```python
from build123d import *

# Parameters (mm, degrees)
SKETCH1_W                    = 20
SKETCH1_H                    = 85
BASE_FLANGE1_DEPTH           = 1.5
EDGE_FLANGE1_DEPTH           = 85
EDGE_FLANGE2_STRIP_W         = 9
EDGE_FLANGE2_STRIP_H         = 1.5
EDGE_FLANGE2_STRIP_CUT_DEPTH = 85
EDGE_FLANGE2_DEPTH           = 85
CUT_EXTRUDE1_DEPTH           = 53.891398166
CUT_EXTRUDE1_DEPTH_BACK      = 53.891398166
SKETCH13_W                   = 25
SKETCH13_H                   = 26.5
CUT_EXTRUDE2_DEPTH           = 53.891398166
CUT_EXTRUDE2_DEPTH_BACK      = 53.891398166
SKETCH14_W                   = 2.598076211
SKETCH14_H                   = 25
SKETCH15_R                   = 2.25
CAGE_MOUNTING_HOLE_DEPTH     = 53.891398166
EDGE_FLANGE3_DEPTH           = 20
ARDUINO_MOUNTING_HOLE_REACH  = 58.065
SKETCH19_R                   = 1.6
FILLET1_R                    = 2.5


# Sheet-metal steps are written as plain solids
with BuildPart() as part:
    # Sketch1 → Base-Flange1 (new body)
    with BuildSketch(Plane(origin=(0, 0, 0), x_dir=(1, 0, 0), z_dir=(0, 1, 0))):
        Rectangle(SKETCH1_W, SKETCH1_H)
    extrude(amount=-BASE_FLANGE1_DEPTH)

    # Edge-Flange1 section (across the edge) → Edge-Flange1 (add)
    with BuildSketch(Plane(origin=(-11.5, 0, -42.5), x_dir=(1, 0, 0), z_dir=(0, 0, 1))):
        with BuildLine():
            Line((-1.5, 1.5), (-1.5, 25))
            Line((-1.5, 25), (0, 25))
            Line((0, 25), (0, 1.5))
            ThreePointArc((0, 1.5), (0.439339828, 0.439339828), (1.5, 0))
            Line((1.5, 0), (1.5, -1.5))
            ThreePointArc((1.5, -1.5), (-0.621320344, -0.621320344), (-1.5, 1.5))
        make_face()
    extrude(amount=EDGE_FLANGE1_DEPTH)

    # Edge-Flange2 strip (across the edge) → Edge-Flange2 strip cut (cut)
    with BuildSketch(Plane(origin=(-11.5, 25, -42.5), x_dir=(0, -1, 0), z_dir=(0, 0, 1))):
        with Locations((-3, -0.75)):
            Rectangle(EDGE_FLANGE2_STRIP_W, EDGE_FLANGE2_STRIP_H)
    extrude(amount=EDGE_FLANGE2_STRIP_CUT_DEPTH, mode=Mode.SUBTRACT)

    # Edge-Flange2 section (across the edge) → Edge-Flange2 (add)
    with BuildSketch(Plane(origin=(-11.5, 25, -42.5), x_dir=(0, -1, 0), z_dir=(0, 0, 1))):
        with BuildLine():
            Line((-1.5, 1.5), (-1.5, 28.5))
            Line((-1.5, 28.5), (0, 28.5))
            Line((0, 28.5), (0, 1.5))
            ThreePointArc((0, 1.5), (0.439339828, 0.439339828), (1.5, 0))
            Line((1.5, 0), (1.5, -1.5))
            ThreePointArc((1.5, -1.5), (-0.621320344, -0.621320344), (-1.5, 1.5))
        make_face()
    extrude(amount=EDGE_FLANGE2_DEPTH)

    # Sketch13 → Cut-Extrude1 (cut, two sides: drawn at the far end of the back side and taken through both)
    with BuildSketch(Plane(origin=(0, 0, 0), x_dir=(0, 0, -1), z_dir=(1, 0, 0)).offset(-CUT_EXTRUDE1_DEPTH_BACK)):
        with Locations((-30, 13.25)):
            Rectangle(SKETCH13_W, SKETCH13_H)
    extrude(amount=CUT_EXTRUDE1_DEPTH + CUT_EXTRUDE1_DEPTH_BACK, mode=Mode.SUBTRACT)

    # Sketch14 → Cut-Extrude2 (cut, two sides: drawn at the far end of the back side and taken through both)
    with BuildSketch(Plane(origin=(0, 0, 0), x_dir=(1, 0, 0), z_dir=(0, 1, 0)).offset(-CUT_EXTRUDE2_DEPTH_BACK)):
        with Locations((-11.299038105, -30)):
            Rectangle(SKETCH14_W, SKETCH14_H)
    extrude(amount=CUT_EXTRUDE2_DEPTH + CUT_EXTRUDE2_DEPTH_BACK, mode=Mode.SUBTRACT)

    # Sketch15 → cage mounting hole (cut, through all)
    with BuildSketch(Plane(origin=(0, 0, 0), x_dir=(1, 0, 0), z_dir=(0, 1, 0))):
        with Locations(Location((0, -35, 0), (0, 0, 270))):
            Circle(SKETCH15_R)
    extrude(amount=-CAGE_MOUNTING_HOLE_DEPTH, mode=Mode.SUBTRACT)

    # Edge-Flange3 section (across the edge) → Edge-Flange3 (add)
    with BuildSketch(Plane(origin=(10, 0, -44), x_dir=(0, 0, 1), z_dir=(-1, 0, 0))):
        with BuildLine():
            Line((-1.5, 1.5), (-1.5, 18.5))
            Line((-1.5, 18.5), (0, 18.5))
            Line((0, 18.5), (0, 1.5))
            ThreePointArc((0, 1.5), (0.439339828, 0.439339828), (1.5, 0))
            Line((1.5, 0), (1.5, -1.5))
            ThreePointArc((1.5, -1.5), (-0.621320344, -0.621320344), (-1.5, 1.5))
        make_face()
    extrude(amount=EDGE_FLANGE3_DEPTH)

    # Sketch19 → arduino mounting hole (cut, up to next)
    with BuildSketch(Plane(origin=(0, 26.5, 0), x_dir=(1, 0, 0), z_dir=(0, 1, 0)), mode=Mode.PRIVATE) as arduino_mounting_hole_sk1:
        with Locations(Location((0.5, 37.5, 0), (0, 0, 180))):
            Circle(SKETCH19_R)
    arduino_mounting_hole_tool1 = extrude(arduino_mounting_hole_sk1.sketch, amount=-ARDUINO_MOUNTING_HOLE_REACH, mode=Mode.PRIVATE) & part.part
    add(arduino_mounting_hole_tool1.solids().sort_by_distance((0.5, 26.5, -37.5))[0], mode=Mode.SUBTRACT)

    # Fillet1
    fillet1_edges = [part.edges().sort_by_distance(p)[0] for p in [
        (10, 18.5, -44.75),
        (-10, 18.5, -44.75),
        (17, 25.75, -42.5),
        (17, 25.75, 17.5),
        (10, -0.75, 42.5),
        (-10, -0.75, 42.5),
    ]]
    fillet(fillet1_edges, radius=FILLET1_R)


solid = part.part
```
The listing builds one solid part. Answer for the finished solid, in the listing's coordinates (mm). A direction names the side the tool comes from. Coordinates: 2 decimals unless noted, no trailing zeros. Loops run counter-clockwise (first coordinate to the right, second up) from the corner with the lowest first, then second, coordinate; pieces in that order, holes last. Notation, with made-up numbers: (54.5, -16) -> (113.5, -16) arc R34 cw to (113.5, 16) -> close; hole circle Ø8 at (22, 20.5). An arc over 180 degrees is marked (long way). Return JSON: item names as keys, results as strings. Group by question number.
(1) A cutting plane is placed at D-D on x = 0. Write down the section's boundary in (y, z), and give its area (3 significant figures).
(2) Find the intervals of material crossed by probe 1 along Z at (x, y) = (0.5, 25.9); probe 2 along Y at (x, z) = (-4.25, 1); probe 3 along X at (y, z) = (-1.1, 35), in increasing order. Write a range as from..to.
(3) Which of the six approach directions +Z, -Z, +X, -X, +Y, -Y give full straight-line access (tool end or side, diameter ignored) to faces 1 (the cylindrical face through (-0.24, 25.76, -38.92)), 2 (the flat face through (0, 0, -1)), 3 (the flat face through (-10, 7, -45))?
(4) Determine the mould class of faces 4 (the cylindrical face through (9, -1, 42)), 5 (the flat face through (0, 10, -45.5)), 6 (the cylindrical face through (-0.86, -0.74, 37.08)), 7 (the flat face through (17, 26, -13)) for opening direction Z: released by +Z, released by -Z, zero draft, split by the parting line, or undercut.
(5) Given pin 1 Ø4 at (y, z) = (1.5, -27.5) entering from +X; pin 2 Ø1.6 at (y, z) = (-0.5, 32.5) entering from -X; pin 3 Ø4 at (y, z) = (7.5, -12.5) entering from +X, each flat-ended and moving along its own axis, determine where each tip first touches the part or whether it passes through.
(6) A cutting plane is placed at C-C on z = 35. Write down the section's boundary in (x, y), and give its area (4 significant figures).
(7) A cutting plane is placed at B-B on y = 17.5. Write down the section's boundary in (x, z).
(8) A cutting plane is placed at A-A on x = -4. Write down the section's boundary in (y, z).
The answers:
{
 "1": {"outline": "(-1.5, -42.5) arc R3 ccw to (1.5, -45.5) -> (18.5, -45.5) -> (18.5, -44) -> (1.5, -44) arc R1.5 cw to (0, -42.5) -> (0, 32.75) -> (-1.5, 32.75) -> close; (-1.5, 37.25) -> (0, 37.25) -> (0, 42.5) -> (-1.5, 42.5) -> close; (25, -42.5) -> (26.5, -42.5) -> (26.5, -39.02) -> (25, -39.02) -> close; (25, -35.98) -> (26.5, -35.98) -> (26.5, 17.5) -> (25, 17.5) -> close", "area": "237 mm^2"},
 "2": {"probe 1": "z = -42.5..-39.1, -35.9..17.5", "probe 2": "y = -1.5..0, 25..26.5", "probe 3": "x = -10..-2.25, 2.25..10"},
 "3": {"face 1": "+Y", "face 2": "+Z, +X", "face 3": "-Z, -X, +Y, -Y"},
 "4": {"face 4": "released by +Z", "face 5": "released by -Z", "face 6": "undercut", "face 7": "zero draft"},
 "5": {"pin 1": "stops at x = 10", "pin 2": "stops at x = -10", "pin 3": "stops at x = -11.5"},
 "6": {"outline": "(-10, -1.5) -> (-2.25, -1.5) -> (-2.25, 0) -> (-10, 0) -> close; (2.25, -1.5) -> (10, -1.5) -> (10, 0) -> (2.25, 0) -> close", "area": "23.25 mm^2"},
 "7": {"outline": "(-13, -42.5) -> (-11.5, -42.5) -> (-11.5, 17.5) -> (-13, 17.5) -> close; (-9.5, -45.5) -> (9.5, -45.5) -> (9.5, -44) -> (-9.5, -44) -> close"},
 "8": {"outline": "(-1.5, -42.5) arc R3 ccw to (1.5, -45.5) -> (18.5, -45.5) -> (18.5, -44) -> (1.5, -44) arc R1.5 cw to (0, -42.5) -> (0, 42.5) -> (-1.5, 42.5) -> close; (25, -42.5) -> (26.5, -42.5) -> (26.5, 17.5) -> (25, 17.5) -> close"}
}
